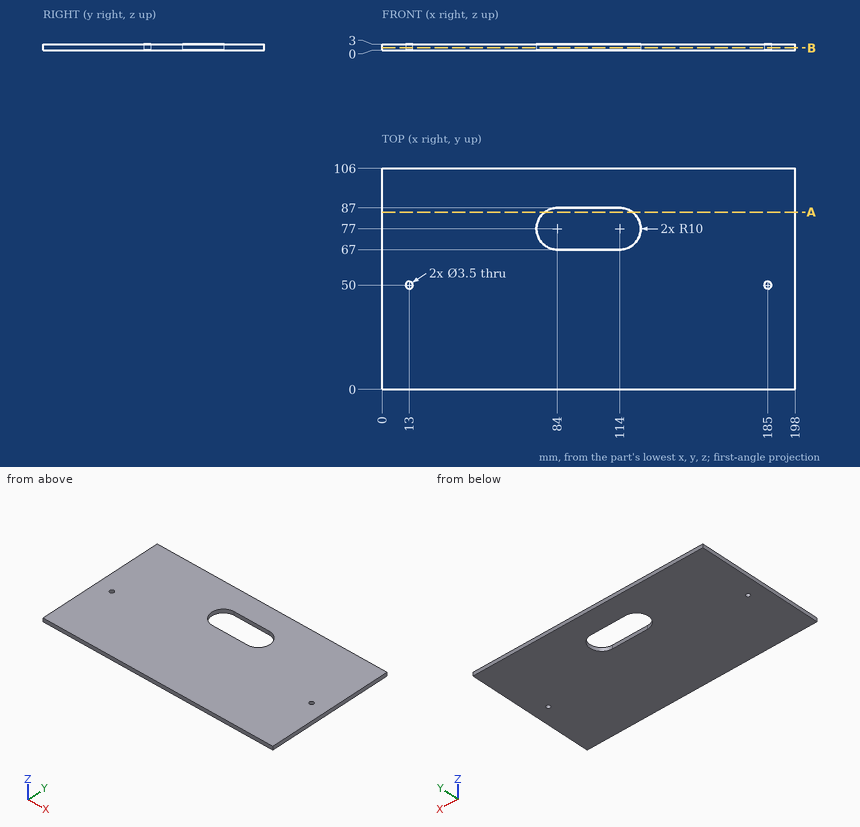
Part print with two shaded views. Sizes in mm from the minimum x, y, z corner. Coordinates: 2 decimals unless noted, no trailing zeros. Order: outer loops, then holes, each group sorted by start corner. A loop starts at its lowest first (then second) coordinate and runs counter-clockwise, first axis right, second up. Notation, with made-up numbers: (-5, 62.25) - (32, 62.25) arc R21 ccw to (32, 87.25) - close; hole circle Ø6 at (27.25, 87.5). An arc over 180 degrees is marked (long way). Write item = value, one per line. Start each with the question number.
1) Saw through at A-A on y = 85. Write the cut outline in (x, z).
2) Flat gauge pin, fed straight in: pin 1 Ø5 at (x, y) = (45, 50) entering from -Z. Where does the tip first touch, or does it go through?
3) Wall check: line 1 along Y through (x, z) = (185, 2.4); line 2 along X through (y, z) = (76.5, 1.05); line 3 along Y through (x, z) = (108.5, 0.95). Give the ranges that are in metal, low to high. Write a range as from..to.
4) Saw through at B-B on z = 1.1. Write the cut outline in (x, y), then the cut area to 3 significant figures.
From the geometry:
q1.outline = (0, 0) - (78, 0) - (78, 3) - (0, 3) - close; (120, 0) - (198, 0) - (198, 3) - (120, 3) - close
q2.pin_1 = 0
q3.line_1 = 0..48.25, 51.75..106
q3.line_2 = 0..74.01, 123.99..198
q3.line_3 = 0..67, 87..106
q4.outline = (0, 0) - (198, 0) - (198, 106) - (0, 106) - close; hole circle Ø3.5 at (13, 50); hole (84, 67) - (114, 67) arc R10 ccw to (114, 87) - (84, 87) arc R10 ccw to start; hole circle Ø3.5 at (185, 50)
q4.area = 20,100 mm^2
